from build123d import *

# Parameters (mm, degrees)
SKETCH1_W           = 25
SKETCH1_H           = 60
BOSS_EXTRUDE1_DEPTH = 3
BOSS_EXTRUDE3_START = -3
SKETCH2_W           = 80
SKETCH2_H           = 40
BOSS_EXTRUDE3_DEPTH = 80
FILLET1_R           = 10
SHELL1_START        = 52
SHELL1_DEPTH        = 38
SKETCH3_R           = 4
CUT_EXTRUDE1_DEPTH  = 100
SKETCH4_R           = 1.75
CUT_EXTRUDE2_DEPTH  = 100
CHAMFER1_SIZE       = 20
FILLET2_R           = 15


with BuildPart() as part:
    # Sketch1 → Boss-Extrude1 (new body)
    with BuildSketch(Plane.XY):
        Rectangle(SKETCH1_W, SKETCH1_H)
        Polygon((12.5, 50), (12.5, 30), (-12.5, 30), (-12.5, 50), (-40, 50), (-40, 90), (40, 90), (40, 50), align=None)
    extrude(amount=BOSS_EXTRUDE1_DEPTH)

    # Sketch2 → Boss-Extrude3 (add)
    with BuildSketch(Plane.XY.offset(3).offset(BOSS_EXTRUDE3_START)):
        with Locations((0, 70)):
            Rectangle(SKETCH2_W, SKETCH2_H)
    extrude(amount=BOSS_EXTRUDE3_DEPTH)

    # Fillet1
    fillet1_edges = [part.edges().sort_by_distance(p)[0] for p in [
        (-40, 70, 80),
        (40, 70, 80),
    ]]
    fillet(fillet1_edges, radius=FILLET1_R)

    # Shell1: read off the stored shape, not the designer's step
    # Shell1 outline → Shell1 (cut)
    with BuildSketch(Plane(origin=(0, 0, 0), x_dir=(1, 0, 0), z_dir=(0, 1, 0)).offset(SHELL1_START)):
        with BuildLine():
            ThreePointArc((30, -78), (35.656854249, -75.656854249), (38, -70))
            Line((38, -70), (38, -2))
            Line((38, -2), (-38, -2))
            Line((-38, -2), (-38, -70))
            ThreePointArc((-38, -70), (-35.656854249, -75.656854249), (-30, -78))
            Line((-30, -78), (30, -78))
        make_face()
    extrude(amount=SHELL1_DEPTH, mode=Mode.SUBTRACT)

    # Sketch3 → Cut-Extrude1 (cut)
    with BuildSketch(Plane(origin=(0, 52, 0), x_dir=(1, 0, 0), z_dir=(0, 1, 0))):
        with Locations(Location((-2, -24.5, 0), (0, 0, 270))):
            Circle(SKETCH3_R)
    extrude(amount=-CUT_EXTRUDE1_DEPTH, mode=Mode.SUBTRACT)

    # Sketch4 → Cut-Extrude2 (cut)
    with BuildSketch(Plane.XY.offset(3)):
        with Locations((-6.75, 25)):
            Circle(SKETCH4_R)
        with Locations((6.75, 25)):
            Circle(SKETCH4_R)
        with Locations((6.75, -25)):
            Circle(SKETCH4_R)
        with Locations((-6.75, -25)):
            Circle(SKETCH4_R)
    extrude(amount=-CUT_EXTRUDE2_DEPTH, mode=Mode.SUBTRACT)

    # Chamfer1
    chamfer1_edges = [part.edges().sort_by_distance(p)[0] for p in [
        (-12.5, 50, 1.5),
        (12.5, 50, 1.5),
    ]]
    chamfer(chamfer1_edges, length=CHAMFER1_SIZE)

    # Fillet2
    fillet2_edges = [part.edges().sort_by_distance(p)[0] for p in [
        (-32.5, 50, 1.5),
        (32.5, 50, 1.5),
        (12.5, 30, 1.5),
        (-12.5, 30, 1.5),
    ]]
    fillet(fillet2_edges, radius=FILLET2_R)


solid = part.part
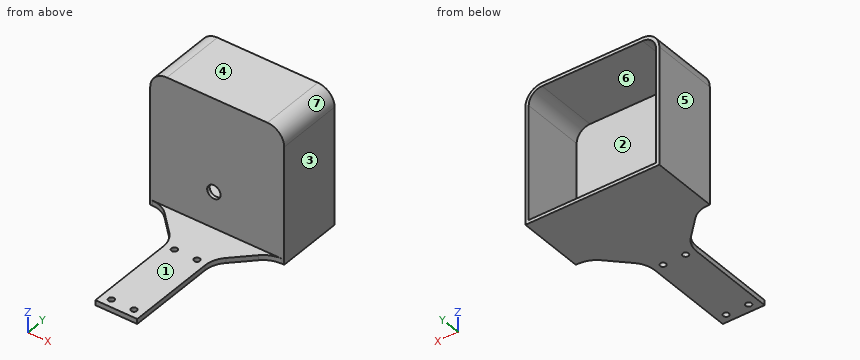
Could you check a few things on this model? Use its own coordinates, in mm. Face numbers are marked on the shaded views. A direction names the side the tool comes from. Coordinates: 2 decimals unless noted, no trailing zeros. Loops run counter-clockwise (first coordinate to the right, second up) from the corner with the lowest first, then second, coordinate; pieces in that order, holes last.
1. Imagine slicing it at C-C (x = -2). Please give me the cut outline in (y, z).
2. Imagine slicing it at B-B (x = 6.75). Please give me the cut outline in (y, z), and give its area (3 significant figures).
3. For the marked faces 1, 2 and 3, which set-ups out of +Z, -Z, +X, -X, +Y, -Y let a thin tool reach every point of the face, with its end or its side?
4. Imagine slicing it at A-A (z = 24.5). Please give me the cut outline in (x, y), and give its area (3 significant figures).
5. For P1, Ø4, axis at x = 9.5, z = 70.5, coming from the +Y side; P2, Ø1, axis at x = -5, z = 45.5, coming from the -Y side; P3, Ø3.5, axis at y = 9.5, z = 1.5, coming from the +X side; P4, Ø2, axis at x = 6.75, y = 25, coming from the +Z side, each with a flat end and sliding along its axis, tell me the tip position at first contact or that it passes through.
6. I need wall thicknesses on L1, parallel to Y at x = 6.75, z = 1.95; L2, parallel to Y at x = -6.75, z = 2.2; L3, parallel to Z at x = 3.5, y = 69. Which ranges of each line are inside material? Lowest first, please.
7. Imagine slicing it at D-D (y = 17.5). Please give me the cut outline in (x, z), and give its area (3 significant figures).
8. We'd pull the mould along X, two halves only. Please class the marked faces 4, 5, 6 and 7: released by +X, released by -X, zero draft, split by the parting line, or undercut.
Computed values:
1. outline: (-30, 0) - (90, 0) - (90, 2) - (52, 2) - (52, 20.5) - (50, 20.5) - (50, 3) - (-30, 3) - close; (50, 28.5) - (52, 28.5) - (52, 78) - (90, 78) - (90, 80) - (50, 80) - close
2. outline: (-30, 0) - (-26.75, 0) - (-26.75, 3) - (-30, 3) - close; (-23.25, 0) - (23.25, 0) - (23.25, 3) - (-23.25, 3) - close; (26.75, 0) - (90, 0) - (90, 2) - (52, 2) - (52, 78) - (90, 78) - (90, 80) - (50, 80) - (50, 3) - (26.75, 3) - close
2. area: 531 mm2
3. face 1: +Z, +X, -X, -Y
3. face 2: +Y
3. face 3: +Z, -Z, +X, +Y, -Y
4. outline: (-40, 50) - (-6, 50) - (-6, 52) - (-38, 52) - (-38, 90) - (-40, 90) - close; (2, 50) - (40, 50) - (40, 90) - (38, 90) - (38, 52) - (2, 52) - close
4. area: 296 mm2
5. P1: stops at y = 52
5. P2: stops at y = 50
5. P3: stops at x = 12.5
5. P4: passes through
6. L1: y = -30 to -26.75, -23.25 to 23.25, 26.75 to 90
6. L2: y = -30 to -26.75, -23.25 to 23.25, 26.75 to 52
6. L3: z = 0 to 2, 78 to 80
7. outline: (-12.5, 0) - (12.5, 0) - (12.5, 3) - (-12.5, 3) - close
7. area: 75.0 mm2
8. face 4: zero draft
8. face 5: released by -X
8. face 6: undercut
8. face 7: released by +X
